The model under review builds one solid part; all positions refer to its coordinate system, in mm. A direction names the side the tool comes from. Coordinates: 2 decimals unless noted, no trailing zeros. Write each loop counter-clockwise with the first axis right and the second up, starting at its lowest first coordinate (ties: lowest second). Pieces come first, ordered by that corner, then holes. Notation, with made-up numbers: M 17,-3 L 31,-3 A19 cw 31,10 Z; hole C -6.75,29.25 d1. An arc over 180 degrees is marked long. Answer as a JSON object with one key per item and string values.
```python
from build123d import *

# Parameters (mm, degrees)
F2_SIZE = 1


with BuildPart() as f1:
    # F0 (on Top) → F1 (revolve)
    with BuildSketch(Plane.XY):
        with BuildLine():
            Line((0, 65.5), (0, 8))
            Line((0, 8), (48, 8))
            Line((48, 8), (48, 65.5))
            ThreePointArc((48, 65.5), (47.56066, 66.56066), (46.5, 67))
            ThreePointArc((46.5, 67), (45.43934, 66.56066), (45, 65.5))
            Line((45, 65.5), (45, 28))
            Line((45, 28), (3, 28))
            Line((3, 28), (3, 65.5))
            ThreePointArc((3, 65.5), (2.56066, 66.56066), (1.5, 67))
            ThreePointArc((1.5, 67), (0.43934, 66.56066), (0, 65.5))
        make_face()
    revolve(axis=Axis((24, 0, 0), (1, 0, 0)))

    # F2
    f2_edges = [f1.edges().sort_by_distance(p)[0] for p in [
        (0, -8, 0),
        (48, -8, 0),
    ]]
    chamfer(f2_edges, length=F2_SIZE)


solid = f1.part
```
(1) For faces 1 (the face through (3, 0.9, -28.2)), 2 (the face through (48, 1, -14)), list the 3-axis set-ups (+Z, -Z, +X, -X, +Y, -Y) from which the entire face can be reached by the end or side of a thin tool; tool diameter is ignored.
Results list:
{"face 1": "none", "face 2": "+Z, -Z, +X, +Y, -Y"}
(2) Add section C-C on x = 32.5. Give the boundary of the cut face in (y, z).
Results list:
{"outline": "C 0,0 d56; hole C 0,0 d16"}
(3) Draft analysis for pull direction Z (two halves, no side actions). For faces 3 (the face through (24.32, -1.73, -7.81)), 4 (the face through (23.706, 25.865, -10.724)), 5 (the face through (0, -1, -14)), state which applies: released by +Z, released by -Z, zero draft, split by the parting line, or undercut.
Results list:
{"face 3": "undercut", "face 4": "split by the parting line", "face 5": "zero draft"}
(4) Add section A-A on z = 0. Give the boundary of the cut face in (x, y).
Results list:
{"outline": "M 0,-65.5 A1.5 ccw 1.5,-67 A1.5 ccw 3,-65.5 L 3,-28 L 45,-28 L 45,-65.5 A1.5 ccw 46.5,-67 A1.5 ccw 48,-65.5 L 48,-9 L 47,-8 L 1,-8 L 0,-9 Z; M 0,9 L 1,8 L 47,8 L 48,9 L 48,65.5 A1.5 ccw 46.5,67 A1.5 ccw 45,65.5 L 45,28 L 3,28 L 3,65.5 A1.5 ccw 1.5,67 A1.5 ccw 0,65.5 Z"}
(5) Wall thickness on line 1 along X through (y, z) = (21.5, -39); line 2 along Z through (x, y) = (17, 0); line 3 along Y through (x, z) = (18, -5) (3 decimals): over which ranges is each line inside the solid? List them lowest first. Write a range as from..to.
Results list:
{"line 1": "0..3, 45..48", "line 2": "-28..-8, 8..28", "line 3": "-27.55..-6.245, 6.245..27.55"}
(6) For pin 1 Ø1 at (x, y) = (39, 23) entering from +Z; pin 2 Ø1 at (x, y) = (22.5, -23.5) entering from +Z, all flat-tipped, find the tip position at first contact; note any pin that passes through.
Results list:
{"pin 1": "z = 16.67", "pin 2": "z = 15.97"}
